Verification items for this drawing (mm, ordinates from the low corner). A direction names the side the tool comes from. Round coordinates to 2 decimals unless told otherwise and drop trailing zeros. Write each loop counter-clockwise with the first axis right and the second up, starting at its lowest first coordinate (ties: lowest second). Pieces come first, ordered by that corner, then holes. Notation, with made-up numbers: M 49.5,23 L 107.5,23 A14 cw 107.5,44 Z; hole C 55.25,31 d4. An arc over 180 degrees is marked long. Write each question's results on one line, items separated by ' | '.
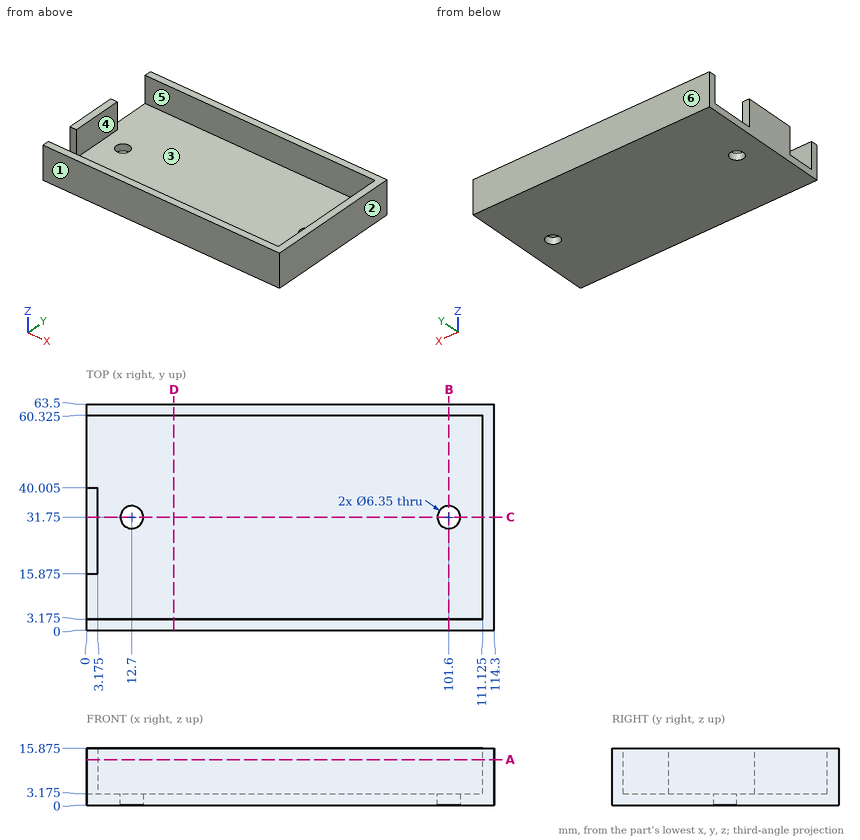
1) Sectioned sample at A-A, the plane z = 12.75. Record the cut outline in (x, y) (3 decimals), and give its area (3 significant figures).
Calculated:
outline: M 0,0 L 114.3,0 L 114.3,63.5 L 0,63.5 L 0,60.325 L 111.125,60.325 L 111.125,3.175 L 0,3.175 Z; M 0,15.875 L 3.175,15.875 L 3.175,40.005 L 0,40.005 Z | area: 984 mm²
2) Draft check along X on the marked faces 1, 2, 3 and 4. Enter one of: pulls with the +X half, pulls with the -X half, needs draft (parallel to the pull), parting line crosses it, or undercut.
Calculated:
face 1: needs draft | face 2: pulls with the +X half | face 3: undercut | face 4: undercut
3) Access from +Z, -Z, +X, -X, +Y, -Y to the whole of each face (thin tool, end or side, straight path). Record for the marked faces 5 and 6.
Calculated:
face 5: +Z, -X | face 6: +Z, -Z, +X, -X, +Y
4) Depth check by flat-ended pin: P1, Ø4, axis at y = 44, z = 2.5, coming from the -X side; P2, Ø6, axis at x = 52, y = 31, coming from the +Z side (3 decimals); P3, Ø5, axis at x = 12.7, y = 31.75, coming from the +Z side. Enter the tip coordinate at first touch or a pass-through.
Calculated:
P1: stops at x = 0 | P2: stops at z = 3.175 | P3: passes through
5) Material ranges on line 1 (X direction, y = 16, z = 9.75) (3 decimals); line 2 (Y direction, x = 101.6, z = 0.85) (3 decimals); line 3 (Y direction, x = 53, z = 13.5) (3 decimals), recorded low to high. Write a range as [from, to].
Calculated:
line 1: x = [0, 3.175], [111.125, 114.3] | line 2: y = [0, 28.575], [34.925, 63.5] | line 3: y = [0, 3.175], [60.325, 63.5]
6) Sectioned sample at C-C, the plane y = 31.75. Record the cut outline in (x, z) (3 decimals).
Calculated:
outline: M 0,0 L 9.525,0 L 9.525,3.175 L 3.175,3.175 L 3.175,15.875 L 0,15.875 Z; M 15.875,0 L 98.425,0 L 98.425,3.175 L 15.875,3.175 Z; M 104.775,0 L 114.3,0 L 114.3,15.875 L 111.125,15.875 L 111.125,3.175 L 104.775,3.175 Z
7) Sectioned sample at D-D, the plane x = 24.5. Record the cut outline in (y, z) (3 decimals), and give its area (3 significant figures).
Calculated:
outline: M 0,0 L 63.5,0 L 63.5,15.875 L 60.325,15.875 L 60.325,3.175 L 3.175,3.175 L 3.175,15.875 L 0,15.875 Z | area: 282 mm²
8) Sectioned sample at B-B, the plane x = 101.6. Record the cut outline in (y, z) (3 decimals).
Calculated:
outline: M 0,0 L 28.575,0 L 28.575,3.175 L 3.175,3.175 L 3.175,15.875 L 0,15.875 Z; M 34.925,0 L 63.5,0 L 63.5,15.875 L 60.325,15.875 L 60.325,3.175 L 34.925,3.175 Z
